Print and shaded views of the part. All mm, measured from the part's lowest x, y and z. Round coordinates to 2 decimals unless told otherwise and drop trailing zeros. Loops run counter-clockwise (first coordinate to the right, second up) from the corner with the lowest first, then second, coordinate; pieces in that order, holes last. Notation, with made-up numbers: (0.5, 26.5) -> (41.5, 26.5) arc R13 cw to (41.5, 30.5) -> close; hole circle Ø7 at (45, 75). An arc over 180 degrees is marked (long way). Answer as CSV lines item,"result".
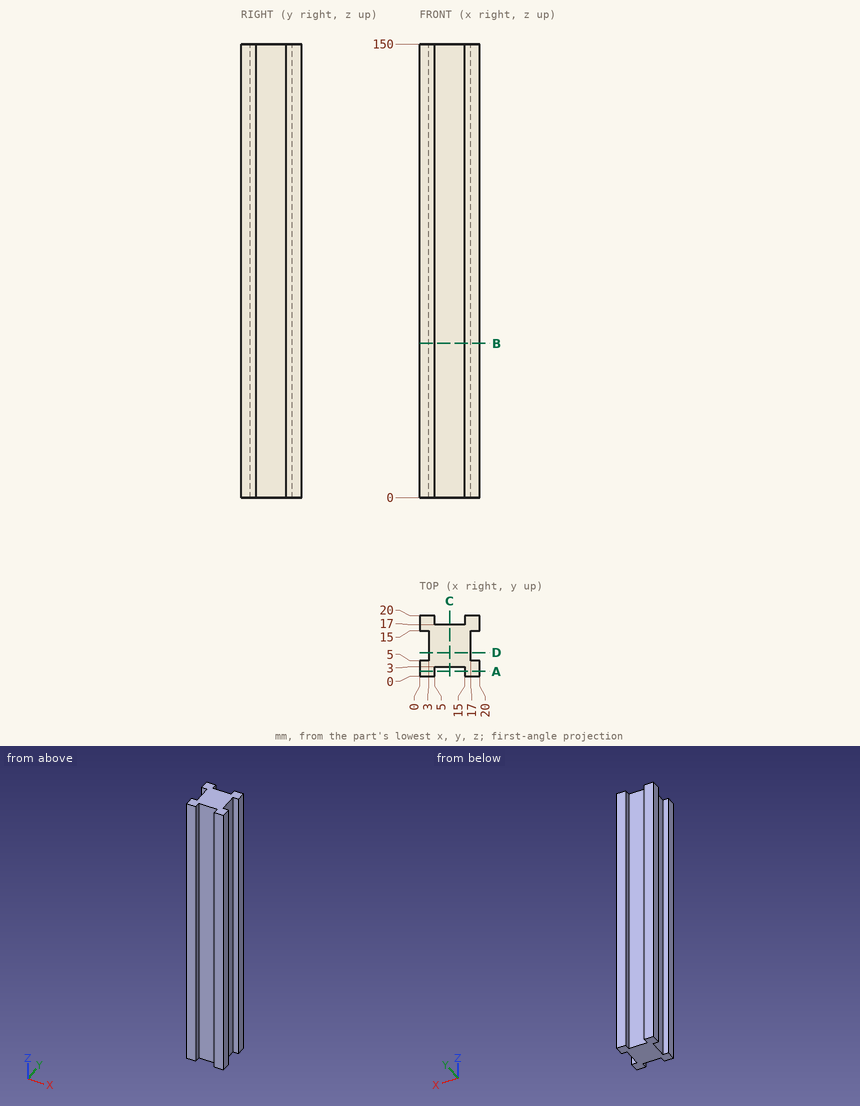
Q1. Saw through at A-A, the plane y = 1.5. Write the cut outline in (x, z), then the cut area to 3 significant figures.
Geometry results:
outline,"(0, 0) -> (5, 0) -> (5, 150) -> (0, 150) -> close; (15, 0) -> (20, 0) -> (20, 150) -> (15, 150) -> close"
area,"1,500 mm2"
Q2. Saw through at C-C, the plane x = 10. Write the cut outline in (y, z).
Geometry results:
outline,"(3, 0) -> (17, 0) -> (17, 150) -> (3, 150) -> close"
Q3. Drill centre lines: line 1 along Y through (x, z) = (19, 7); line 2 along X through (y, z) = (9, 27.5). Where is each one in solid material? Low to high.
Geometry results:
line 1,"0 to 5, 15 to 20"
line 2,"3 to 17"
Q4. Saw through at B-B, the plane z = 51. Write the cut outline in (x, y).
Geometry results:
outline,"(0, 0) -> (5, 0) -> (5, 3) -> (15, 3) -> (15, 0) -> (20, 0) -> (20, 5) -> (17, 5) -> (17, 15) -> (20, 15) -> (20, 20) -> (15, 20) -> (15, 17) -> (5, 17) -> (5, 20) -> (0, 20) -> (0, 15) -> (3, 15) -> (3, 5) -> (0, 5) -> close"
Q5. Drop flat-ended pins along their axis: P1, Ø3, axis at x = 12.5, z = 82.5, coming from the +Y side; P2, Ø1.5, axis at y = 10, z = 74.5, coming from the +X side; P3, Ø5, axis at x = 9.5, z = 51.5, coming from the -Y side. Give the stop position or say it passes through.
Geometry results:
P1,"y = 17"
P2,"x = 17"
P3,"y = 3"
